Geometry check sheet. Reference: the model listing, model coordinates, mm. A direction names the side the tool comes from. Round coordinates to 2 decimals unless told otherwise and drop trailing zeros. Loops run counter-clockwise (first coordinate to the right, second up) from the corner with the lowest first, then second, coordinate; pieces in that order, holes last. Notation, with made-up numbers: M 87,-31 L 142,-31 A24 ccw 142,-3 Z; hole C 45.5,-16.5 d7. An arc over 180 degrees is marked long. Use one line per item in the form item = value. Start each with the question number.
1. Cross-section at C-C (x = 2.5). State how many separate pieces and enclosed holes the cut face has, then the cut area to 3 significant figures.
2. Material ranges on line 1 (Y direction, x = -9.45, z = -21.1); line 2 (Y direction, x = 2.5, z = -42.75); line 3 (Z direction, x = -9.45, y = 15), recorded low to high.
3. Go/stop test with flat-tipped pins: pin 1 (4 mm diameter, centred on x = 9.5, y = 13.5, fed in from +Z); pin 2 (14.5 mm diameter, centred on x = 2.5, y = 15, fed in from +Z); pin 3 (5 mm diameter, centred on y = 15, z = -21.1, fed in from -X). Record where each tip stops, or that it passes through.
4. Draft check along Y on faces 1 (the cylindrical face through (0.245, -29.145, -55.301)), 2 (the cylindrical face through (0.081, 18.794, -0.236)), 3 (the cylindrical face through (-0.245, 29.145, -55.301)). Enter one of: pulls with the +Y half, pulls with the -Y half, needs draft (parallel to the pull), parting line crosses it, or undercut.
5. Cross-section at A-A (z = 37). Record the boundary of the cut face in (x, y).
6. Set-up check for faces 4 (the cylindrical face through (-4.05, 13.52, -20.49)), 5 (the flat face through (-4, -11, 45.873)), 6 (the conical face through (5.7, -22.8, -50.8)): record each of +Z, -Z, +X, -X, +Y, -Y from which the full face is reachable in a straight line by a thin tool's end or side.
```python
from build123d import *

# Parameters (mm, degrees)
BLOCK_SKETCH_W                                 = 112.406774914
BLOCK_SKETCH_H                                 = 60
BLOCK_DEPTH                                    = 17.5
F_3_8_NPT_FLOW_CONNECTOR_AT_2_COUNT            = 2
F_3_8_NPT_FLOW_CONNECTOR_AT_2_PITCH            = 30
F_1_8_NPT_PRESSURE_SENSOR_CONNECTOR_AT_2_COUNT = 2
F_1_8_NPT_PRESSURE_SENSOR_CONNECTOR_AT_2_PITCH = 42.2
F_1_8_NPT_PRESSURE_SENSOR_CONNECTOR_AT_3_COUNT = 2
F_1_8_NPT_PRESSURE_SENSOR_CONNECTOR_AT_3_PITCH = 51.776828794
F_1_8_NPT_PRESSURE_SENSOR_CONNECTOR_AT_4_COUNT = 2
F_1_8_NPT_PRESSURE_SENSOR_CONNECTOR_AT_4_PITCH = 30
PRESSURE_SENSOR_HOLE_REACH                     = 37
SKETCH11_R                                     = 1.6
M8X1_0_TAPPED_HOLE1_D                          = 7
M10X1_0_TAPPED_HOLE1_D                         = 9
ROUNDED_EDGES_R                                = 3


with BuildPart() as part:
    # block_sketch → block (new body, symmetric)
    with BuildSketch(Plane(origin=(0, 0, 0), x_dir=(0, 0, -1), z_dir=(1, 0, 0))):
        Rectangle(BLOCK_SKETCH_W, BLOCK_SKETCH_H)
    extrude(amount=BLOCK_DEPTH, both=True)

    # Sketch6 → 3/8 NPT_flow_connector (revolve, cut)
    with BuildSketch(Plane(origin=(2.5, 15, 56.203387457), x_dir=(0, -1, 0), z_dir=(1, 0, 0))):
        Polygon((0, 0), (0, 21.668582582), (7.1374, 17.38), (7.1374, 10.33), (8.282218717, 10.33), (8.5725, 0.635), (9.2075, 0), align=None)
    f_3_8_npt_flow_connector = revolve(axis=Axis((2.5, 15, 62.553387457), (0, 0, -1)), mode=Mode.SUBTRACT)

    # 3/8 NPT_flow_connector at 2: 3/8 NPT_flow_connector ×2
    with Locations(*[(0, -i * F_3_8_NPT_FLOW_CONNECTOR_AT_2_PITCH, 0) for i in range(1, F_3_8_NPT_FLOW_CONNECTOR_AT_2_COUNT)]):
        add(f_3_8_npt_flow_connector, mode=Mode.SUBTRACT)

    # Sketch15 → M8_flow_channel (revolve, cut)
    with BuildSketch(Plane(origin=(2.5, -15, 56.203387457), x_dir=(0, -1, 0), z_dir=(1, 0, 0))):
        Polygon((0, 0), (0, 42.018852388), (6.35, 38.203387457), (6.35, 0), align=None)
    m8_flow_channel = revolve(axis=Axis((2.5, -15, 62.553387457), (0, 0, -1)), mode=Mode.SUBTRACT)

    # Sketch20 → M10_flow_channel (revolve, cut)
    with BuildSketch(Plane(origin=(2.5, 15, 56.203387457), x_dir=(0, -1, 0), z_dir=(1, 0, 0))):
        Polygon((0, 0), (0, 42.018852388), (6.35, 38.203387457), (6.35, 0), align=None)
    m10_flow_channel = revolve(axis=Axis((2.5, 15, 62.553387457), (0, 0, -1)), mode=Mode.SUBTRACT)

    # flow_mirror: M10_flow_channel, 3/8 NPT_flow_connector, M8_flow_channel across plane
    add(m10_flow_channel.mirror(Plane.XY), mode=Mode.SUBTRACT)
    add(f_3_8_npt_flow_connector.mirror(Plane.XY), mode=Mode.SUBTRACT)
    add(m8_flow_channel.mirror(Plane.XY), mode=Mode.SUBTRACT)

    # flow_mirror copy 1 sketch → flow_mirror copy 1 (revolve, cut)
    with BuildSketch(Plane(origin=(2.5, -15, -56.203387457), x_dir=(0, -1, 0), z_dir=(1, 0, 0))):
        Polygon((0, 0), (0, -21.668582582), (7.1374, -17.38), (7.1374, -10.33), (8.282218717, -10.33), (8.5725, -0.635), (9.2075, 0), align=None)
    revolve(axis=Axis((2.5, -15, -62.553387457), (0, 0, -1)), mode=Mode.SUBTRACT)

    # Sketch4 → 1/8 NPT_pressure_sensor_connector (revolve, cut)
    with BuildSketch(Plane(origin=(-17.5, -15, 21.1), x_dir=(0, 0, 1), z_dir=(0, 1, 0))):
        Polygon((0, 0), (0, 14.153468714), (4.2164, 11.62), (4.2164, 6.92), (4.955191683, 6.92), (5.143373, 0.635), (5.778373, 0), align=None)
    f_1_8_npt_pressure_sensor_connector = revolve(axis=Axis((-23.85, -15, 21.1), (1, 0, 0)), mode=Mode.SUBTRACT)

    # 1/8 NPT_pressure_sensor_connector at 2: 1/8 NPT_pressure_sensor_connector ×2
    with Locations(*[(0, 0, -i * F_1_8_NPT_PRESSURE_SENSOR_CONNECTOR_AT_2_PITCH) for i in range(1, F_1_8_NPT_PRESSURE_SENSOR_CONNECTOR_AT_2_COUNT)]):
        add(f_1_8_npt_pressure_sensor_connector, mode=Mode.SUBTRACT)

    # 1/8 NPT_pressure_sensor_connector at 3: 1/8 NPT_pressure_sensor_connector ×2
    with Locations(*[Vector(0, 0.579409761, -0.815036397) * (i * F_1_8_NPT_PRESSURE_SENSOR_CONNECTOR_AT_3_PITCH) for i in range(1, F_1_8_NPT_PRESSURE_SENSOR_CONNECTOR_AT_3_COUNT)]):
        add(f_1_8_npt_pressure_sensor_connector, mode=Mode.SUBTRACT)

    # 1/8 NPT_pressure_sensor_connector at 4: 1/8 NPT_pressure_sensor_connector ×2
    with Locations(*[(0, i * F_1_8_NPT_PRESSURE_SENSOR_CONNECTOR_AT_4_PITCH, 0) for i in range(1, F_1_8_NPT_PRESSURE_SENSOR_CONNECTOR_AT_4_COUNT)]):
        add(f_1_8_npt_pressure_sensor_connector, mode=Mode.SUBTRACT)

    # Sketch11 → pressure_sensor_hole (cut, up to next)
    with BuildSketch(Plane(origin=(-17.5, 14.596917944, 0), x_dir=(0, -1, 0), z_dir=(1, 0, 0)), mode=Mode.PRIVATE) as pressure_sensor_hole_sk1:
        with Locations((29.596917944, 21.1)):
            Circle(SKETCH11_R)
    pressure_sensor_hole_tool1 = extrude(pressure_sensor_hole_sk1.sketch, amount=PRESSURE_SENSOR_HOLE_REACH, mode=Mode.PRIVATE) & part.part
    add(pressure_sensor_hole_tool1.solids().sort_by_distance((-17.5, -15, -21.1))[0], mode=Mode.SUBTRACT)
    # Sketch11 → pressure_sensor_hole (cut, up to next)
    with BuildSketch(Plane(origin=(-17.5, 14.596917944, 0), x_dir=(0, -1, 0), z_dir=(1, 0, 0)), mode=Mode.PRIVATE) as pressure_sensor_hole_sk2:
        with Locations((29.596917944, -21.1)):
            Circle(SKETCH11_R)
    pressure_sensor_hole_tool2 = extrude(pressure_sensor_hole_sk2.sketch, amount=PRESSURE_SENSOR_HOLE_REACH, mode=Mode.PRIVATE) & part.part
    add(pressure_sensor_hole_tool2.solids().sort_by_distance((-17.5, -15, 21.1))[0], mode=Mode.SUBTRACT)
    # Sketch11 → pressure_sensor_hole (cut, up to next)
    with BuildSketch(Plane(origin=(-17.5, 14.596917944, 0), x_dir=(0, -1, 0), z_dir=(1, 0, 0)), mode=Mode.PRIVATE) as pressure_sensor_hole_sk3:
        with Locations((-0.403082056, 21.1)):
            Circle(SKETCH11_R)
    pressure_sensor_hole_tool3 = extrude(pressure_sensor_hole_sk3.sketch, amount=PRESSURE_SENSOR_HOLE_REACH, mode=Mode.PRIVATE) & part.part
    add(pressure_sensor_hole_tool3.solids().sort_by_distance((-17.5, 15, -21.1))[0], mode=Mode.SUBTRACT)
    # Sketch11 → pressure_sensor_hole (cut, up to next)
    with BuildSketch(Plane(origin=(-17.5, 14.596917944, 0), x_dir=(0, -1, 0), z_dir=(1, 0, 0)), mode=Mode.PRIVATE) as pressure_sensor_hole_sk4:
        with Locations((-0.403082056, -21.1)):
            Circle(SKETCH11_R)
    pressure_sensor_hole_tool4 = extrude(pressure_sensor_hole_sk4.sketch, amount=PRESSURE_SENSOR_HOLE_REACH, mode=Mode.PRIVATE) & part.part
    add(pressure_sensor_hole_tool4.solids().sort_by_distance((-17.5, 15, 21.1))[0], mode=Mode.SUBTRACT)

    # M8x1.0 Tapped Hole1 (through all)
    with Locations(Plane.XY.offset(56.203387457)):
        with Locations((2.5, -15)):
            Hole(M8X1_0_TAPPED_HOLE1_D / 2)

    # M10x1.0 Tapped Hole1 (through all)
    with Locations(Plane.XY.offset(56.203387457)):
        with Locations((2.5, 15)):
            Hole(M10X1_0_TAPPED_HOLE1_D / 2)

    # rounded_edges
    rounded_edges_edges = [part.edges().sort_by_distance(p)[0] for p in [
        (0, 30, 56.203387457),
        (0, 30, -56.203387457),
        (0, -30, -56.203387457),
        (0, -30, 56.203387457),
    ]]
    fillet(rounded_edges_edges, radius=ROUNDED_EDGES_R)


solid = part.part
```
Reported:
q1.separate_pieces = 3
q1.enclosed_holes = 0
q1.area = 3,990 mm²
q2.line_1 = -30 to -19.22, -10.78 to 10.78, 19.22 to 30
q2.line_2 = -30 to -22.14, -7.86 to 7.86, 22.14 to 30
q2.line_3 = -56.2 to -25.32, -16.88 to 16.88, 25.32 to 56.2
q3.pin_1 = 56.15
q3.pin_2 = 45.87
q3.pin_3 = -4.85
q4.face_1 = pulls with the -Y half
q4.face_2 = undercut
q4.face_3 = pulls with the +Y half
q5.outline = M -17.5,-30 L 17.5,-30 L 17.5,30 L -17.5,30 Z; hole C 2.5,-15 d12.7; hole C 2.5,15 d12.7
q6.face_4 = -X
q6.face_5 = +Z
q6.face_6 = -Z
